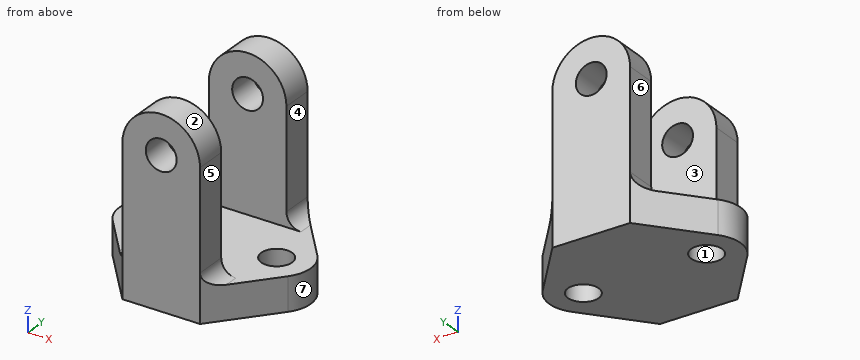
from build123d import *

# Parameters (mm, degrees)
SKETCH1_W                      = 41.4
SKETCH1_H                      = 33.02
SKETCH1_R                      = 3.175
BOSS_EXTRUDE1_DEPTH            = 12
SKETCH2_W                      = 41.4
SKETCH2_H                      = 6.51
BOSS_EXTRUDE2_DEPTH            = 53
CUT_EXTRUDE1_REACH             = 72.186
SKETCH4_R                      = 3.175
CUT_EXTRUDE1_DIRECTION_2_REACH = 72.186
CUT_EXTRUDE3_REACH             = 72.186
CUT_EXTRUDE3_DIRECTION_2_REACH = 72.186
CUT_EXTRUDE4_DEPTH             = 12
BOSS_EXTRUDE3_DEPTH            = 12
FILLET3_R                      = 3
CUT_EXTRUDE5_DEPTH             = 5.08


with BuildPart() as part:
    # Sketch1 → Boss-Extrude1 (new body)
    with BuildSketch(Plane.XY):
        Rectangle(SKETCH1_W, SKETCH1_H)
        with Locations((12.7, 0)):
            Circle(SKETCH1_R, mode=Mode.SUBTRACT)
        with Locations((-12.7, 0)):
            Circle(SKETCH1_R, mode=Mode.SUBTRACT)
    extrude(amount=BOSS_EXTRUDE1_DEPTH)

    # Sketch2 → Boss-Extrude2 (add)
    with BuildSketch(Plane.XY.offset(12)):
        with Locations((0, 13.255)):
            Rectangle(SKETCH2_W, SKETCH2_H)
        with Locations((0, -13.255)):
            Rectangle(SKETCH2_W, SKETCH2_H)
    extrude(amount=BOSS_EXTRUDE2_DEPTH)

    # Cut-Extrude1: up to this face of the body (flat: up to its plane)
    cut_extrude1_end = Plane(part.part.faces().sort_by_distance((0, -16.51, 32.5))[0])
    # Sketch4 → Cut-Extrude1 (cut, up to the picked face)
    with BuildSketch(Plane(origin=(0, 0, 0), x_dir=(1, 0, 0), z_dir=(0, 1, 0)), mode=Mode.PRIVATE) as cut_extrude1_sk1:
        with Locations(Location((0, -35.5, 0), (0, 0, 270))):
            Circle(SKETCH4_R)
    cut_extrude1_tool1 = split(extrude(cut_extrude1_sk1.sketch, amount=-CUT_EXTRUDE1_REACH, mode=Mode.PRIVATE), bisect_by=cut_extrude1_end, keep=Keep.BOTH, mode=Mode.PRIVATE)
    add(cut_extrude1_tool1.solids().sort_by(Axis((0, 0, 35.5), (0, -1, 0)))[0], mode=Mode.SUBTRACT)

    # Cut-Extrude1 direction 2: up to this face of the body (flat: up to its plane)
    cut_extrude1_direction_2_end = Plane(part.part.faces().sort_by_distance((0, 16.51, 32.5))[0])
    # Sketch4 → Cut-Extrude1 direction 2 (cut, up to the picked face)
    with BuildSketch(Plane(origin=(0, 0, 0), x_dir=(1, 0, 0), z_dir=(0, 1, 0)), mode=Mode.PRIVATE) as cut_extrude1_direction_2_sk1:
        with Locations(Location((0, -35.5, 0), (0, 0, 270))):
            Circle(SKETCH4_R)
    cut_extrude1_direction_2_tool1 = split(extrude(cut_extrude1_direction_2_sk1.sketch, amount=CUT_EXTRUDE1_DIRECTION_2_REACH, mode=Mode.PRIVATE), bisect_by=cut_extrude1_direction_2_end, keep=Keep.BOTH, mode=Mode.PRIVATE)
    add(cut_extrude1_direction_2_tool1.solids().sort_by(Axis((0, 0, 35.5), (0, 1, 0)))[0], mode=Mode.SUBTRACT)

    # Cut-Extrude3: up to this face of the body (flat: up to its plane)
    cut_extrude3_end = Plane(part.part.faces().sort_by_distance((-19.929353518, -16.51, 32.5))[0])
    # Sketch6 → Cut-Extrude3 (cut, up to the picked face)
    with BuildSketch(Plane(origin=(0, 0, 0), x_dir=(1, 0, 0), z_dir=(0, 1, 0)), mode=Mode.PRIVATE) as cut_extrude3_sk1:
        with BuildLine():
            Line((-8, -35.5), (-8, -20))
            Line((-8, -20), (-8, -12))
            Line((-8, -12), (-16, -12))
            Line((-16, -12), (-20.7, -12))
            Line((-20.7, -12), (-20.7, -65))
            Line((-20.7, -65), (20.7, -65))
            Line((20.7, -65), (20.7, -12))
            Line((20.7, -12), (16, -12))
            Line((16, -12), (8, -12))
            Line((8, -12), (8, -20))
            Line((8, -20), (8, -35.5))
            ThreePointArc((8, -35.5), (0, -43.5), (-8, -35.5))
        make_face()
    cut_extrude3_tool1 = split(extrude(cut_extrude3_sk1.sketch, amount=-CUT_EXTRUDE3_REACH, mode=Mode.PRIVATE), bisect_by=cut_extrude3_end, keep=Keep.BOTH, mode=Mode.PRIVATE)
    add(cut_extrude3_tool1.solids().sort_by(Axis((-8.67253, 0, 27.75), (0, -1, 0)))[0], mode=Mode.SUBTRACT)

    # Cut-Extrude3 direction 2: up to this face of the body (flat: up to its plane)
    cut_extrude3_direction_2_end = Plane(part.part.faces().sort_by_distance((19.929353518, 16.51, 32.5))[0])
    # Sketch6 → Cut-Extrude3 direction 2 (cut, up to the picked face)
    with BuildSketch(Plane(origin=(0, 0, 0), x_dir=(1, 0, 0), z_dir=(0, 1, 0)), mode=Mode.PRIVATE) as cut_extrude3_direction_2_sk1:
        with BuildLine():
            Line((-8, -35.5), (-8, -20))
            Line((-8, -20), (-8, -12))
            Line((-8, -12), (-16, -12))
            Line((-16, -12), (-20.7, -12))
            Line((-20.7, -12), (-20.7, -65))
            Line((-20.7, -65), (20.7, -65))
            Line((20.7, -65), (20.7, -12))
            Line((20.7, -12), (16, -12))
            Line((16, -12), (8, -12))
            Line((8, -12), (8, -20))
            Line((8, -20), (8, -35.5))
            ThreePointArc((8, -35.5), (0, -43.5), (-8, -35.5))
        make_face()
    cut_extrude3_direction_2_tool1 = split(extrude(cut_extrude3_direction_2_sk1.sketch, amount=CUT_EXTRUDE3_DIRECTION_2_REACH, mode=Mode.PRIVATE), bisect_by=cut_extrude3_direction_2_end, keep=Keep.BOTH, mode=Mode.PRIVATE)
    add(cut_extrude3_direction_2_tool1.solids().sort_by(Axis((-8.67253, 0, 27.75), (0, 1, 0)))[0], mode=Mode.SUBTRACT)

    # Sketch7 → Cut-Extrude4 (cut)
    with BuildSketch(Plane.XY):
        with BuildLine():
            ThreePointArc((-12.7, 7), (-19.7, 0), (-12.7, -7))
            Line((-12.7, -7), (-8, -7))
            Line((-8, -7), (-8, -16.51))
            Line((-8, -16.51), (-20.7, -16.51))
            Line((-20.7, -16.51), (-20.7, 16.51))
            Line((-20.7, 16.51), (-8, 16.51))
            Line((-8, 16.51), (-8, 7))
            Line((-8, 7), (-12.7, 7))
        make_face()
        with BuildLine():
            Line((12.7, 7), (8, 7))
            Line((8, 7), (8, 16.51))
            Line((8, 16.51), (20.7, 16.51))
            Line((20.7, 16.51), (20.7, -16.51))
            Line((20.7, -16.51), (8, -16.51))
            Line((8, -16.51), (8, -7))
            Line((8, -7), (12.7, -7))
            ThreePointArc((12.7, -7), (19.7, 0), (12.7, 7))
        make_face()
    extrude(amount=CUT_EXTRUDE4_DEPTH, mode=Mode.SUBTRACT)

    # Sketch8 → Boss-Extrude3 (add)
    with BuildSketch(Plane.XY):
        with BuildLine():
            Line((8, -16.51), (18.065759147, -4.495400847))
            ThreePointArc((18.065759147, -4.495400847), (15.660759537, -6.343020019), (12.7, -7))
            Line((12.7, -7), (8, -7))
            Line((8, -7), (8, -16.51))
        make_face()
        with BuildLine():
            ThreePointArc((-18.065759147, -4.495400847), (-15.660759537, -6.343020019), (-12.7, -7))
            Line((-12.7, -7), (-8, -7))
            Line((-8, -7), (-8, -16.51))
            Line((-8, -16.51), (-18.065759147, -4.495400847))
        make_face()
        with BuildLine():
            Line((8, 16.51), (18.065759147, 4.495400847))
            ThreePointArc((18.065759147, 4.495400847), (15.660759537, 6.343020019), (12.7, 7))
            Line((12.7, 7), (8, 7))
            Line((8, 7), (8, 16.51))
        make_face()
        with BuildLine():
            Line((-8, 16.51), (-18.065759147, 4.495400847))
            ThreePointArc((-18.065759147, 4.495400847), (-15.660759537, 6.343020019), (-12.7, 7))
            Line((-12.7, 7), (-8, 7))
            Line((-8, 7), (-8, 16.51))
        make_face()
    extrude(amount=BOSS_EXTRUDE3_DEPTH)

    # Fillet3
    fillet3_edges = [part.edges().sort_by_distance(p)[0] for p in [
        (8, -13.255, 12),
        (-8, -13.255, 12),
        (8, 13.255, 12),
        (-8, 13.255, 12),
    ]]
    fillet(fillet3_edges, radius=FILLET3_R)

    # Sketch10 → Cut-Extrude5 (cut)
    with BuildSketch(Plane.XY):
        with BuildLine():
            Line((-8, 16.51), (-18.065759147, 4.495400847))
            ThreePointArc((-18.065759147, 4.495400847), (-19.7, 0), (-18.065759147, -4.495400847))
            Line((-18.065759147, -4.495400847), (-8, -16.51))
            Line((-8, -16.51), (8, -16.51))
            Line((8, -16.51), (18.065759147, -4.495400847))
            ThreePointArc((18.065759147, -4.495400847), (19.7, 0), (18.065759147, 4.495400847))
            Line((18.065759147, 4.495400847), (8, 16.51))
            Line((8, 16.51), (-8, 16.51))
        make_face()
    extrude(amount=CUT_EXTRUDE5_DEPTH, mode=Mode.SUBTRACT)


solid = part.part
Work out the finished part from the listing and answer in its coordinate system (mm). Face numbers are marked on the shaded views. A direction names the side the tool comes from. Coordinates: 2 decimals unless noted, no trailing zeros. Loops run counter-clockwise (first coordinate to the right, second up) from the corner with the lowest first, then second, coordinate; pieces in that order, holes last. Notation, with made-up numbers: (-11.5, -4.75) -> (35.5, -4.75) arc R17 ccw to (35.5, 4.25) -> close; hole circle Ø11 at (70, 71.5). An arc over 180 degrees is marked (long way). Answer as CSV lines item,"result".
1) The part is cut by section A-A (z = 31.5). Give the vertices of the cut face in (x, y), and give its area (3 significant figures).
A:
outline,"(-8, -16.51) -> (8, -16.51) -> (8, -10) -> (-8, -10) -> close; (-8, 10) -> (8, 10) -> (8, 16.51) -> (-8, 16.51) -> close"
area,"208 mm²"
2) Flat-ended cylindrical pins translate along their axes: pin 1 (5 mm diameter, centred on y = 13, z = 25, fed in from +X); pin 2 (3.5 mm diameter, centred on y = 13, z = 20.5, fed in from -X); pin 3 (7.5 mm diameter, centred on x = -12.7, y = 0, fed in from -Z); pin 4 (5.5 mm diameter, centred on x = 0, z = 35.5, fed in from -Y). Find the tip coordinate at first contact, or state that the pin passes through.
A:
pin 1,"stops at x = 8"
pin 2,"stops at x = -8"
pin 3,"stops at z = 5.08"
pin 4,"passes through"
3) For the marked faces 5, 6 and 7, determine the directions among +Z, -Z, +X, -X, +Y, -Y from which every point of the face is accessible in a straight line to the end or side of a thin tool.
A:
face 5,"+Z, +X, +Y, -Y"
face 6,"+Z, -X, +Y, -Y"
face 7,"+Z, -Z, +X"
4) For a pull along X with two mould halves and no side action, classify the marked faces 1, 2, 3 and 4 as released by +X, released by -X, zero draft, split by the parting line, or undercut.
A:
face 1,"undercut"
face 2,"split by the parting line"
face 3,"zero draft"
face 4,"released by +X"
5) The part is cut by section D-D (y = 0). Give the vertices of the cut face in (x, z) (3 decimals).
A:
outline,"(-19.7, 5.08) -> (-15.875, 5.08) -> (-15.875, 12) -> (-19.7, 12) -> close; (-9.525, 5.08) -> (9.525, 5.08) -> (9.525, 12) -> (-9.525, 12) -> close; (15.875, 5.08) -> (19.7, 5.08) -> (19.7, 12) -> (15.875, 12) -> close"
6) The part is cut by section B-B (x = 0). Give the vertices of the cut face in (y, z) (3 decimals), and give its area (3 significant figures).
A:
outline,"(-16.51, 5.08) -> (16.51, 5.08) -> (16.51, 32.325) -> (10, 32.325) -> (10, 12) -> (-10, 12) -> (-10, 32.325) -> (-16.51, 32.325) -> close; (-16.51, 38.675) -> (-10, 38.675) -> (-10, 43.5) -> (-16.51, 43.5) -> close; (10, 38.675) -> (16.51, 38.675) -> (16.51, 43.5) -> (10, 43.5) -> close"
area,"556 mm²"
7) Straight lines are drawn through the part: probe 1 along Z at (x, y) = (0, 13) (3 decimals); probe 2 along Y at (x, z) = (-5, 19.5); probe 3 along X at (y, z) = (-14, 35.5) (3 decimals). For each, find the intervals that lie inside material, in ascending order.
A:
probe 1,"z = 5.08 to 32.325, 38.675 to 43.5"
probe 2,"y = -16.51 to -10, 10 to 16.51"
probe 3,"x = -8 to -3.175, 3.175 to 8"
8) The part is cut by section C-C (z = 10). Give the vertices of the cut face in (x, y) (3 decimals), and give its area (3 significant figures).
A:
outline,"(-18.066, -4.495) -> (-8, -16.51) -> (8, -16.51) -> (18.066, -4.495) arc R7 ccw to (18.066, 4.495) -> (8, 16.51) -> (-8, 16.51) -> (-18.066, 4.495) arc R7 ccw to start; hole circle Ø6.35 at (-12.7, 0); hole circle Ø6.35 at (12.7, 0)"
area,"908 mm²"
